from build123d import *

# Parameters (mm, degrees)
SKETCH_2_R               = 3.6
EXTRUDE_1_DEPTH          = 1.2
SKETCH_3_R               = 1
EXTRUDE_2_DEPTH          = 1.2
PATTERN_CIRCULAR_2_COUNT = 4


with BuildPart() as part:
    # 草圖2 → 伸長1 (new body)
    with BuildSketch(Plane.XY):
        Circle(SKETCH_2_R)
    extrude(amount=EXTRUDE_1_DEPTH)

    # 草圖3 → 伸長2 (add)
    with BuildSketch(Plane(origin=(0, 0, 0), x_dir=(-1, 0, 0), z_dir=(0, 0, -1))):
        with Locations(Location((0, 0, 0), (0, 0, 180))):
            Circle(SKETCH_3_R)
    extrude(amount=EXTRUDE_2_DEPTH)

    # 草圖4 → 除料-疊層拉伸1 section 0
    with BuildSketch(Plane.XY.offset(1.2), mode=Mode.PRIVATE) as loft_1_s0:
        with BuildLine():
            Line((-0.25, 2.9), (0.25, 2.9))
            Line((0.25, 2.9), (0.25, -2.9))
            Line((0.25, -2.9), (-0.25, -2.9))
            Line((-0.25, -2.9), (-0.25, 2.9))
        make_face()
    loft_1 = loft([loft_1_s0.sketch, Vertex(0, 0, 0)], mode=Mode.SUBTRACT)

    # 環狀複製排列2: 除料-疊層拉伸1 ×4 about axis
    pattern_circular_2_axis = Axis((0, 0, 0), (0, 0, 1))
    for i in range(1, PATTERN_CIRCULAR_2_COUNT):
        add(loft_1.rotate(pattern_circular_2_axis, i * 360 / PATTERN_CIRCULAR_2_COUNT), mode=Mode.SUBTRACT)


solid = part.part
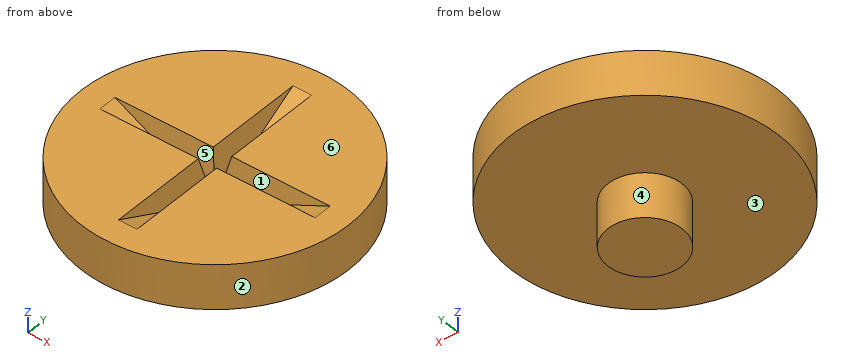
Input: part model. Units: mm. Frame: model coordinates. Face numbers are marked on the shaded views. A direction names the side the tool comes from. Give positions to 0.01 mm unless a question says otherwise; leave off trailing zeros. Write each loop counter-clockwise with the first axis right and the second up, starting at its lowest first coordinate (ties: lowest second). Pieces come first, ordered by that corner, then holes. Notation, with made-up numbers: (5.5, 66) -> (35.5, 66) arc R23 ccw to (35.5, 79) -> close; hole circle Ø1 at (-5.75, -28). An arc over 180 degrees is marked (long way). Use one line per item in the form item = value. Start each with the question number.
1) Set-up query: the marked faces 1, 2 and 3. Return all of +Z, -Z, +X, -X, +Y, -Y with unobstructed straight access to the full face (end or side cutting, diameter ignored); none if empty.
2) Pin query (flat end, axial travel): pin 1 (1 mm diameter, centred on x = -2.5, z = 0, fed in from -Y); pin 2 (4 mm diameter, centred on x = -3, y = 1.5, fed in from -Z). Return the tip coordinate at first contact, or that it passes through.
3) Ray query, probe 1 along Y at (x, z) = (0, 0.25); probe 2 along Z at (x, y) = (1.75, 0.5); probe 3 along Y at (x, z) = (2, 0.4). Return the intervals inside material, ascending. Write a range as from..to.
4) Section query A-A on z = 0.1. Return the cut outline in (x, y), then the cut area to 3 significant figures.
5) Draft query along Y for the marked faces 4, 5 and 6. Return one class per face: pulls with the +Y half, pulls with the -Y half, needs draft (parallel to the pull), parting line crosses it, or undercut.
6) Section query C-C on x = -2. Return the cut outline in (y, z), then the cut area to 3 significant figures.
7) Section query B-B on y = 1.75. Return the cut outline in (x, z), then the cut area to 3 significant figures.
8) Section query D-D on z = -0.45. Return the cut outline in (x, y).
Outcome:
q1.face_1 = +Z
q1.face_2 = +Z, -Z
q1.face_3 = -Z
q2.pin_1 = -2.99
q2.pin_2 = 0
q3.probe_1 = -3.6..-0.6, 0.6..3.6
q3.probe_2 = 0..1.2
q3.probe_3 = -2.99..2.99
q4.outline = circle Ø7.2 at (0, 0); hole (-0.24, -0.02) -> (-0.02, -0.02) -> (-0.02, -0.24) -> (0.02, -0.24) -> (0.02, -0.02) -> (0.24, -0.02) -> (0.24, 0.02) -> (0.02, 0.02) -> (0.02, 0.24) -> (-0.02, 0.24) -> (-0.02, 0.02) -> (-0.24, 0.02) -> close
q4.area = 40.7 mm^2
q5.face_4 = parting line crosses it
q5.face_5 = undercut
q5.face_6 = needs draft
q6.outline = (-2.99, 0) -> (2.99, 0) -> (2.99, 1.2) -> (0.25, 1.2) -> (0.17, 0.83) -> (-0.17, 0.83) -> (-0.25, 1.2) -> (-2.99, 1.2) -> close
q6.area = 7.03 mm^2
q7.outline = (-3.15, 0) -> (3.15, 0) -> (3.15, 1.2) -> (0.25, 1.2) -> (0.15, 0.72) -> (-0.15, 0.72) -> (-0.25, 1.2) -> (-3.15, 1.2) -> close
q7.area = 7.36 mm^2
q8.outline = circle Ø2 at (0, 0)
